```python
from build123d import *

# Parameters (mm, degrees)
F1_DEPTH = 203.2
F3_W     = 12.7
F3_H     = 1143
F4_DEPTH = 203.201


with BuildPart() as f1:
    # F0 (on Front) → F1 (new body)
    with BuildSketch(Plane.XZ):
        Polygon((101.6, 1574.8), (0, 1828.8), (-101.6, 1574.8), (-50.8, 1574.8), (-152.4, 1320.8), (-101.6, 1320.8), (-243.84, 965.2), (-177.8, 965.2), (-360.68, 508), (-254, 508), (-457.2, 0), (457.2, 0), (254, 508), (360.68, 508), (177.8, 965.2), (243.84, 965.2), (101.6, 1320.8), (152.4, 1320.8), (50.8, 1574.8), align=None)
    extrude(amount=F1_DEPTH)

    # F3 (on face) → F4 (cut, through all)
    with BuildSketch(Plane.XZ.offset(203.2)):
        with Locations((0, 1333.5)):
            Rectangle(F3_W, F3_H)
    extrude(amount=-F4_DEPTH, mode=Mode.SUBTRACT)


solid = f1.part
```
Geometry check sheet. Reference: the model listing, model coordinates, mm. A direction names the side the tool comes from. Coordinates: 2 decimals unless noted, no trailing zeros. Order: outer loops, then holes, each group sorted by start corner. A loop starts at its lowest first (then second) coordinate and runs counter-clockwise, first axis right, second up. Notation, with made-up numbers: (62.25, 0.5) - (82.25, 0.5) arc R31 ccw to (82.25, 26.5) - close; hole circle Ø1 at (-32.75, 51.5). An arc over 180 degrees is marked (long way). Use one line per item in the form item = value.
1. Section check A-A (z = 797.5). Record the boundary of the cut face in (x, y).
Here are the results:
outline = (-244.88, -203.2) - (-6.35, -203.2) - (-6.35, 0) - (-244.88, 0) - close; (6.35, -203.2) - (244.88, -203.2) - (244.88, 0) - (6.35, 0) - close
2. Section check D-D (x = 396). Record the boundary of the cut face in (y, z), then the cut area to 3 significant figures.
Here are the results:
outline = (-203.2, 0) - (0, 0) - (0, 153) - (-203.2, 153) - close
area = 31,100 mm²
3. Scan lines: line 1 (X direction, y = -32, z = 1284.5); line 2 (X direction, y = -21, z = 1330); line 3 (X direction, y = -163.5, z = 149.5). Record each from-to range of solid material in increasing order.
Here are the results:
line_1 = -116.12 to -6.35, 6.35 to 116.12
line_2 = -148.72 to -6.35, 6.35 to 148.72
line_3 = -397.4 to 397.4
4. Gauge pin test, flat ends, axial feed: pin 1 (10 mm diameter, centred on y = -115, z = 949.5, fed in from -X); pin 2 (6 mm diameter, centred on y = -148.5, z = 942.5, fed in from +X); pin 3 (4 mm diameter, centred on x = 3, y = -149.5, fed in from +Z). Record the tip position at first contact, or that the pin passes through.
Here are the results:
pin_1 = -186.08
pin_2 = 188.08
pin_3 = 762
5. Section check C-C (y = -142.5). Record the boundary of the cut face in (x, z) (3 decimals).
Here are the results:
outline = (-457.2, 0) - (457.2, 0) - (254, 508) - (360.68, 508) - (177.8, 965.2) - (243.84, 965.2) - (101.6, 1320.8) - (152.4, 1320.8) - (50.8, 1574.8) - (101.6, 1574.8) - (6.35, 1812.925) - (6.35, 762) - (-6.35, 762) - (-6.35, 1812.925) - (-101.6, 1574.8) - (-50.8, 1574.8) - (-152.4, 1320.8) - (-101.6, 1320.8) - (-243.84, 965.2) - (-177.8, 965.2) - (-360.68, 508) - (-254, 508) - close
6. Section check B-B (x = 196.5). Record the boundary of the cut face in (y, z), then the cut area to 3 significant figures.
Here are the results:
outline = (-203.2, 0) - (0, 0) - (0, 918.45) - (-203.2, 918.45) - close; (-203.2, 965.2) - (0, 965.2) - (0, 1083.55) - (-203.2, 1083.55) - close
area = 211,000 mm²
7. Access from +Z, -Z, +X, -X, +Y, -Y to the whole of each face (thin tool, end or side, straight path). Record for faces 1 (the face through (-53.31, -100.18, 1695.53)), 2 (the face through (-127, -100, 1320.8)), 3 (the face through (-6.35, -103, 1280)), 4 (the face through (270.52, -100.18, 733.4)).
Here are the results:
face_1 = +Z, -X, +Y, -Y
face_2 = -X, +Y, -Y
face_3 = +Z, +Y, -Y
face_4 = +X, +Y, -Y
